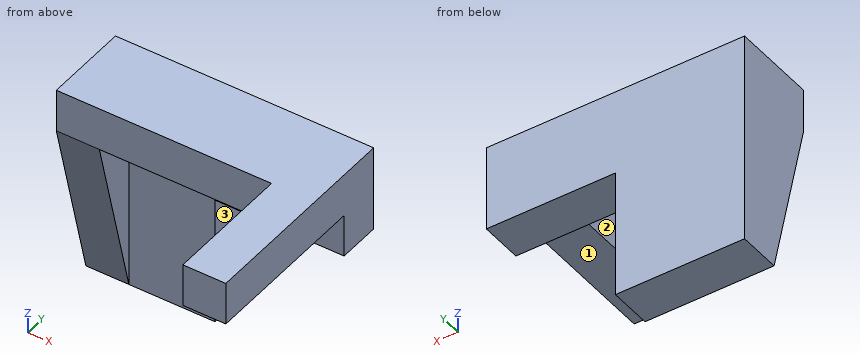
```python
from build123d import *

# Parameters (mm, degrees)
F1_DEPTH  = 1270
F2_W      = 508
F2_H      = 762
F3_DEPTH  = 1016
F4_W      = 1270
F4_H      = 254
F5_DEPTH  = 1016
F7_DEPTH  = 254.001
F8_W      = 762
F8_H      = 762
F9_DEPTH  = 254.001
F10_W     = 508
F10_H     = 254
F11_DEPTH = 762
F12_W     = 254
F12_H     = 762
F13_DEPTH = 1016.001
F15_DEPTH = 254.001


with BuildPart() as f1:
    # F0 (on Front) → F1 (new body)
    with BuildSketch(Plane.XZ):
        Polygon((0, 1270), (0, 0), (762, 0), (762, 762), (1524, 762), (1524, 1270), align=None)
    extrude(amount=F1_DEPTH)

    # F2 (on face) → F3 (cut)
    with BuildSketch(Plane.XZ.offset(1270)):
        with Locations((508, 381)):
            Rectangle(F2_W, F2_H)
    extrude(amount=-F3_DEPTH, mode=Mode.SUBTRACT)

    # F4 (on face) → F5 (cut)
    with BuildSketch(Plane.XZ.offset(1270)):
        with Locations((889, 889)):
            Rectangle(F4_W, F4_H)
    extrude(amount=-F5_DEPTH, mode=Mode.SUBTRACT)

    # F6 (on face) → F7 (cut, through all)
    with BuildSketch(Plane.YZ.offset(254)):
        Polygon((-254, 0), (-1270, 1016), (-1270, 0), align=None)
    extrude(amount=-F7_DEPTH, mode=Mode.SUBTRACT)

    # F8 (on face) → F9 (cut, through all)
    with BuildSketch(Plane(origin=(0, 0, 1016), x_dir=(1, 0, 0), z_dir=(0, 0, -1))):
        with Locations((889, 889)):
            Rectangle(F8_W, F8_H)
    extrude(amount=-F9_DEPTH, mode=Mode.SUBTRACT)

    # F10 (on face) → F11 (cut)
    with BuildSketch(Plane.XZ.offset(1270)):
        with Locations((254, 1143)):
            Rectangle(F10_W, F10_H)
    extrude(amount=-F11_DEPTH, mode=Mode.SUBTRACT)

    # F12 (on face) → F13 (cut, through all)
    with BuildSketch(Plane.XY.offset(1016)):
        with Locations((127, -889)):
            Rectangle(F12_W, F12_H)
    extrude(amount=-F13_DEPTH, mode=Mode.SUBTRACT)

    # F14 (on face) → F15 (cut, through all)
    with BuildSketch(Plane.YZ.offset(254)):
        Polygon((-254, 0), (-508, 1016), (-508, 254), align=None)
    extrude(amount=-F15_DEPTH, mode=Mode.SUBTRACT)


solid = f1.part
```
Source: CAD feature listing. Evaluate the final solid. Frame: model axes, mm. Face numbers are marked on the shaded views. A direction names the side the tool comes from. Round coordinates to 2 decimals unless told otherwise and drop trailing zeros. Loops run counter-clockwise (first coordinate to the right, second up) from the corner with the lowest first, then second, coordinate; pieces in that order, holes last.
1. Section query B-B on y = -375.5. Output: boundary loops of the cut face in (x, z), and give its area (3 significant figures).
2. Access query for the marked faces 1, 2 and 3. Directions: +Z, -Z, +X, -X, +Y, -Y. A direction counts if a zero-diameter tool reaches every point of the face in a straight line with its end or side. Return the directions, or none.
3. Contact query for flat-ended pins moving along their axis: pin 1 (1.5 mm diameter, centred on y = -678, z = 1079, fed in from -X); pin 2 (1.5 mm diameter, centred on x = 1353.5, z = 828.5, fed in from -Y). Output: stop coordinate, or through.
4. Section query D-D on y = -635. Output: boundary loops of the cut face in (x, z), and give its area (3 significant figures).
5. Ray query, L1, parallel to Z at x = 799, y = -189.5; L2, parallel to Y at x = 757, z = 327.5; L3, parallel to Y at x = 754, z = 1120.5. Return the intervals inside material, ascending.
6. Section query A-A on z = 611. Output: boundary loops of the cut face in (x, y).
7. Section query C-C on x = 115. Output: boundary loops of the cut face in (y, z).
Answers below:
1. outline: (0, 486) - (254, 486) - (254, 1016) - (1524, 1016) - (1524, 1270) - (0, 1270) - close
1. area: 522,000 mm2
2. face 1: -Z, +X, -Y
2. face 2: +Z, -Z, -X, -Y
2. face 3: -Z, +X, +Y, -Y
3. pin 1: stops at x = 1270
3. pin 2: stops at y = -254
4. outline: (1270, 1016) - (1524, 1016) - (1524, 1270) - (1270, 1270) - close
4. area: 64,500 mm2
5. L1: z = 762 to 1270
5. L2: y = -254 to 0
5. L3: y = -508 to 0
6. outline: (0, -406.75) - (254, -406.75) - (254, -254) - (762, -254) - (762, 0) - (0, 0) - close
7. outline: (-508, 1016) - (-254, 0) - (0, 0) - (0, 1270) - (-508, 1270) - close
